Design review of the part built by this model. Coordinates are the model's own, in mm. Face numbers are marked on the shaded views. Give positions to 0.01 mm unless a question says otherwise; leave off trailing zeros. Order: outer loops, then holes, each group sorted by start corner. A loop starts at its lowest first (then second) coordinate and runs counter-clockwise, first axis right, second up. Notation, with made-up numbers: (34.5, -22) -> (86.5, -22) arc R19 cw to (86.5, -6) -> close; hole circle Ø3 at (19, 47.5). An arc over 180 degrees is marked (long way). One line per item, written item: value. Start each with the question number.
1) Consider section D-D (x = -12). State the section outline as (y, z) points.
2) Wall thickness on line 1 along X through (y, z) = (3.85, 12); line 2 along Z through (x, y) = (0, 0.9); line 3 along X through (y, z) = (3.45, -19): over which ranges is each line inside the solid? List them lowest first. Write a range as from..to.
3) For pin 1 (1 mm diameter, centred on x = -16.5, y = 2.5, fed in from -Z); pin 2 (1 mm diameter, centred on y = 0.5, z = -4, fed in from +X), all flat-tipped, find the tip position at first contact; note any pin that passes through.
4) Consider section C-C (y = 0.9). State how many separate pieces and enclosed holes the cut face has, plus the area to 3 significant figures.
5) Consider section A-A (z = 0). State the section outline as (x, y) points.
6) The part is to be moulded in two halves that separate along Z. For the marked faces 1, 2 and 3, say which applies: released by +Z, released by -Z, zero draft, split by the parting line, or undercut.
7) Consider section B-B (x = 0). State the section outline as (y, z) points, plus the area to 3 significant figures.
from build123d import *

# Parameters (mm, degrees)
SKETCH_1_R      = 1.25
SKETCH_1_R_2    = 16
EXTRUDE_1_DEPTH = 4.5
SKETCH_2_R      = 16
SKETCH_2_R_2    = 15.5
EXTRUDE_2_DEPTH = 0.5


with BuildPart() as part:
    # 草图1 → 凸台-拉伸1 (new body)
    with BuildSketch(Plane(origin=(0, 0, 0), x_dir=(1, 0, 0), z_dir=(0, 1, 0))):
        with BuildLine():
            ThreePointArc((21.75410191, -2.433747417), (23, 0), (21.75410191, 2.433747417))
            ThreePointArc((21.75410191, 2.433747417), (19.021130326, 6.180339887), (19.029958982, 10.81779726))
            ThreePointArc((19.029958982, 10.81779726), (18.607390871, 13.519060803), (16.168917304, 14.7556833))
            ThreePointArc((16.168917304, 14.7556833), (11.755705046, 16.180339887), (9.037018527, 19.937311066))
            ThreePointArc((9.037018527, 19.937311066), (7.107390871, 21.874299875), (4.407755848, 21.44144969))
            ThreePointArc((4.407755848, 21.44144969), (0, 20), (-4.407755848, 21.44144969))
            ThreePointArc((-4.407755848, 21.44144969), (-7.107390871, 21.874299875), (-9.037018527, 19.937311066))
            ThreePointArc((-9.037018527, 19.937311066), (-11.755705046, 16.180339887), (-16.168917304, 14.7556833))
            ThreePointArc((-16.168917304, 14.7556833), (-18.607390871, 13.519060803), (-19.029958982, 10.81779726))
            ThreePointArc((-19.029958982, 10.81779726), (-19.021130326, 6.180339887), (-21.75410191, 2.433747417))
            ThreePointArc((-21.75410191, 2.433747417), (-23, 0), (-21.75410191, -2.433747417))
            ThreePointArc((-21.75410191, -2.433747417), (-19.021130326, -6.180339887), (-19.029958982, -10.81779726))
            ThreePointArc((-19.029958982, -10.81779726), (-18.607390871, -13.519060803), (-16.168917304, -14.7556833))
            ThreePointArc((-16.168917304, -14.7556833), (-11.755705046, -16.180339887), (-9.037018527, -19.937311066))
            ThreePointArc((-9.037018527, -19.937311066), (-7.107390871, -21.874299875), (-4.407755848, -21.44144969))
            ThreePointArc((-4.407755848, -21.44144969), (0, -20), (4.407755848, -21.44144969))
            ThreePointArc((4.407755848, -21.44144969), (7.107390871, -21.874299875), (9.037018527, -19.937311066))
            ThreePointArc((9.037018527, -19.937311066), (11.755705046, -16.180339887), (16.168917304, -14.7556833))
            ThreePointArc((16.168917304, -14.7556833), (18.607390871, -13.519060803), (19.029958982, -10.81779726))
            ThreePointArc((19.029958982, -10.81779726), (19.021130326, -6.180339887), (21.75410191, -2.433747417))
        make_face()
        with Locations((20, 0)):
            Circle(SKETCH_1_R, mode=Mode.SUBTRACT)
        with Locations((16.180339887, -11.755705046)):
            Circle(SKETCH_1_R, mode=Mode.SUBTRACT)
        with Locations((6.180339887, -19.021130326)):
            Circle(SKETCH_1_R, mode=Mode.SUBTRACT)
        with Locations((-6.180339887, -19.021130326)):
            Circle(SKETCH_1_R, mode=Mode.SUBTRACT)
        with Locations((-16.180339887, -11.755705046)):
            Circle(SKETCH_1_R, mode=Mode.SUBTRACT)
        with Locations((-20, 0)):
            Circle(SKETCH_1_R, mode=Mode.SUBTRACT)
        with Locations((-16.180339887, 11.755705046)):
            Circle(SKETCH_1_R, mode=Mode.SUBTRACT)
        with Locations((-6.180339887, 19.021130326)):
            Circle(SKETCH_1_R, mode=Mode.SUBTRACT)
        with Locations((6.180339887, 19.021130326)):
            Circle(SKETCH_1_R, mode=Mode.SUBTRACT)
        with Locations((16.180339887, 11.755705046)):
            Circle(SKETCH_1_R, mode=Mode.SUBTRACT)
        Circle(SKETCH_1_R_2, mode=Mode.SUBTRACT)
    extrude(amount=EXTRUDE_1_DEPTH)

    # 草图2 → 凸台-拉伸2 (add)
    with BuildSketch(Plane(origin=(0, 4.5, 0), x_dir=(1, 0, 0), z_dir=(0, 1, 0))):
        Circle(SKETCH_2_R)
        Circle(SKETCH_2_R_2, mode=Mode.SUBTRACT)
    extrude(amount=-EXTRUDE_2_DEPTH)


solid = part.part
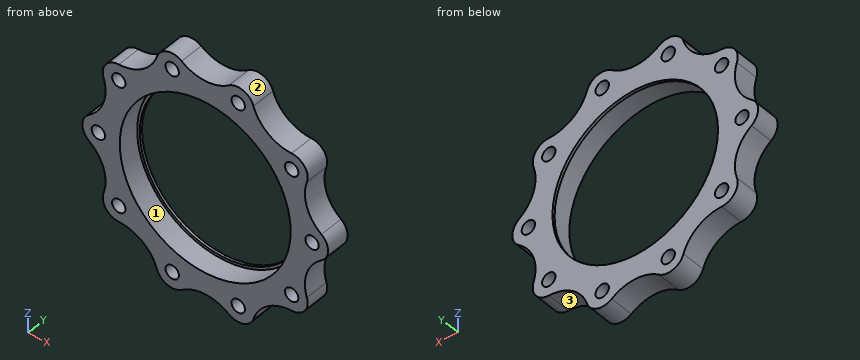
Checked values:
1. outline: (0, -16.01) -> (4.5, -16.01) -> (4.5, -9.81) -> (4, -9.81) -> (4, -10.58) -> (0, -10.58) -> close; (0, 10.58) -> (4, 10.58) -> (4, 9.81) -> (4.5, 9.81) -> (4.5, 16.01) -> (0, 16.01) -> close
2. line 1: x = -19.17..-17.41, -14.95..-10.58, 10.58..14.95, 17.41..19.17
2. line 2: z = -20..-16, 16..20
2. line 3: x = -9.41..-7.43, -4.93..4.93, 7.43..9.41
3. pin 1: stops at z = -14.76
3. pin 2: stops at x = 20.57
4. separate pieces: 1
4. enclosed holes: 11
4. area: 577 mm^2
5. outline: (-23, 0) -> (-21.25, 0) -> (-21.25, 4.5) -> (-23, 4.5) -> close; (-18.75, 0) -> (-16, 0) -> (-16, 4) -> (-15.5, 4) -> (-15.5, 4.5) -> (-18.75, 4.5) -> close; (15.5, 4) -> (16, 4) -> (16, 0) -> (18.75, 0) -> (18.75, 4.5) -> (15.5, 4.5) -> close; (21.25, 0) -> (23, 0) -> (23, 4.5) -> (21.25, 4.5) -> close
6. face 1: undercut
6. face 2: released by +Z
6. face 3: released by -Z
7. outline: (0, -20) -> (4.5, -20) -> (4.5, -15.5) -> (4, -15.5) -> (4, -16) -> (0, -16) -> close; (0, 16) -> (4, 16) -> (4, 15.5) -> (4.5, 15.5) -> (4.5, 20) -> (0, 20) -> close
7. area: 36.5 mm^2
